from build123d import *

# Parameters (mm, degrees)
ESBO_O1_W                  = 50
ESBO_O1_H                  = 50
ESBO_O1_W_2                = 46
ESBO_O1_H_2                = 46
RESSALTO_EXTRUS_O1_DEPTH   = 1000
CORTE_EXTRUS_O1_DEPTH      = 1002.561281201
CORTE_EXTRUS_O1_DEPTH_BACK = 1002.561281201
ESBO_O2_R                  = 5


with BuildPart() as part:
    # Esboço1 → Ressalto-extrusão1 (new body)
    with BuildSketch(Plane(origin=(0, 0, 0), x_dir=(1, 0, 0), z_dir=(0, 1, 0))):
        Rectangle(ESBO_O1_W, ESBO_O1_H)
        Rectangle(ESBO_O1_W_2, ESBO_O1_H_2, mode=Mode.SUBTRACT)
    extrude(amount=RESSALTO_EXTRUS_O1_DEPTH)

    # Esboço2 → Corte-extrusão1 (cut, two sides: drawn at the far end of the back side and taken through both)
    with BuildSketch(Plane.XY.offset(25).offset(-CORTE_EXTRUS_O1_DEPTH_BACK)):
        with Locations(Location((0, 970, 0), (0, 0, 180))):
            Circle(ESBO_O2_R)
    extrude(amount=CORTE_EXTRUS_O1_DEPTH + CORTE_EXTRUS_O1_DEPTH_BACK, mode=Mode.SUBTRACT)


solid = part.part
CAD build for the part. Positions are in the model's coordinates, mm. A direction names the side the tool comes from. Coordinates: 2 decimals unless noted, no trailing zeros. Loops run counter-clockwise (first coordinate to the right, second up) from the corner with the lowest first, then second, coordinate; pieces in that order, holes last. Notation, with made-up numbers: (-29.5, 73) - (-5.5, 73) arc R20 ccw to (-5.5, 100) - close; hole circle Ø9 at (77, 29.25). An arc over 180 degrees is marked (long way). Write item = value, one per line. Start each with the question number.
Q1. Pull direction X, two halves, no side cores. Call faces 3 (the flat face through (0, 493, -23)), 4 (the flat face through (-2, 0, 24)), 5 (the flat face through (-25, 493, 0)): pulls with the +X half, pulls with the -X half, needs draft (parallel to the pull), parting line crosses it, or undercut.
Q2. Flat gauge pins, fed straight in: pin 1 Ø16 at (x, y) = (0, 970) entering from +Z; pin 2 Ø8 at (x, z) = (-5, -18.5) entering from -Y. Where does each tip first touch, or does it go through?
Q3. Cut at A-A, the plane z = 9. List the corners of the cut face in (x, y).
Q4. Which spindle directions (+Z, -Z, +X, -X, +Y, -Y) get a long thin tool onto all of the face, cutting with end or side? Do faces 1 (the flat face through (-23, 493, 0)), 2 (the flat face through (-2, 1000, 24)). Say none if no direction does.
Q5. Cut at B-B, the plane x = -15.5. List the corners of the cut face in (y, z), then the cut area to 3 significant figures.
Q6. Cut at C-C, the plane y = 937. List the corners of the cut face in (x, z), then the cut area to 3 significant figures.
Q7. Drill centre lines: L1, parallel to X at y = 435, z = -16; L2, parallel to Y at x = 0, z = 24.4. Where is each one in solid material? Low to high.
Computed:
q1.face_3 = undercut
q1.face_4 = needs draft
q1.face_5 = pulls with the -X half
q2.pin_1 = 25
q2.pin_2 = through
q3.outline = (-25, 0) - (-23, 0) - (-23, 1000) - (-25, 1000) - close; (23, 0) - (25, 0) - (25, 1000) - (23, 1000) - close
q4.face_1 = +Y, -Y
q4.face_2 = +Z, -Z, +X, -X, +Y
q5.outline = (0, -25) - (1000, -25) - (1000, -23) - (0, -23) - close; (0, 23) - (1000, 23) - (1000, 25) - (0, 25) - close
q5.area = 4,000 mm²
q6.outline = (-25, -25) - (25, -25) - (25, 25) - (-25, 25) - close; hole (-23, -23) - (23, -23) - (23, 23) - (-23, 23) - close
q6.area = 384 mm²
q7.L1 = -25 to -23, 23 to 25
q7.L2 = 0 to 965, 975 to 1000
